Build history of the part. All positions in model axes, mm. Face numbers are marked on the shaded views. A direction names the side the tool comes from. Round coordinates to 2 decimals unless told otherwise and drop trailing zeros. Loops run counter-clockwise (first coordinate to the right, second up) from the corner with the lowest first, then second, coordinate; pieces in that order, holes last.
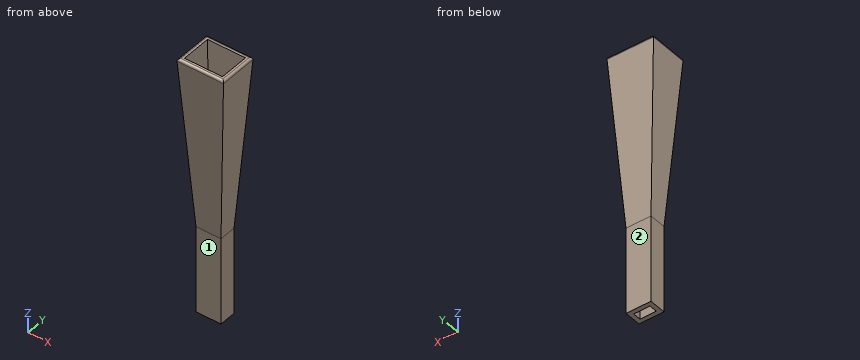
Autodesk Inventor part; units mm, degrees
ref_plane "Endebene" through (0, 0, 59.75) normal (0, 0, 1) x (1, 0, 0)
ref_plane "YZ Plane" through (0, 0, 0) normal (1, 0, 0) x (0, 1, 0)
ref_plane "XZ Plane" through (0, 0, 0) normal (0, 1, 0) x (-1, 0, 0)
sketch "Skizze1" plane through (0, 0, 0) normal (0, 0, 1) x (1, 0, 0)
  line L0 (1.8795, 0.94) -> (-1.8795, 0.94)
  line L1 (-1.8795, 0.94) -> (-1.8795, -0.94)
  line L2 (-1.8795, -0.94) -> (1.8795, -0.94)
  line L3 (1.8795, -0.94) -> (1.8795, 0.94)
  line L4 (1.8795, 0.94) -> (-1.8795, -0.94) construction
  line L5 (-1.8795, 0.94) -> (1.8795, -0.94) construction
  line L6 (-2.8795, -1.94) -> (-2.8795, 1.94)
  line L7 (-2.8795, 1.94) -> (2.8795, 1.94)
  line L8 (2.8795, 1.94) -> (2.8795, -1.94)
  line L9 (2.8795, -1.94) -> (-2.8795, -1.94)
  point P0 (0, 0)
  dimension "d0" = 1.88
  dimension "d1" = 3.759
  dimension "d2" = 1
extrude "Ex1-RWG" add sketch "Skizze1" along normal blind 20
ref_plane "Endebene" through (0, 0, 59.75) normal (0, 0, 1) x (1, 0, 0)
sketch "S-Hornöffnung" plane through (0, 0, 59.75) normal (0, 0, 1) x (1, 0, 0)
  line L0 (2.8795, -1.94) -> (2.8795, 1.94)
  line L1 (2.8795, 1.94) -> (-2.8795, 1.94)
  line L2 (-2.8795, 1.94) -> (-2.8795, -1.94)
  line L3 (-2.8795, -1.94) -> (2.8795, -1.94)
  line L4 (1.8795, 0.94) -> (1.8795, -0.94)
  line L5 (1.8795, -0.94) -> (-1.8795, -0.94)
  line L6 (-1.8795, -0.94) -> (-1.8795, 0.94)
  line L7 (-1.8795, 0.94) -> (1.8795, 0.94)
  line L8 (4.3795, 3.44) -> (4.3795, -3.44)
  line L9 (4.3795, -3.44) -> (-4.3795, -3.44)
  line L10 (-4.3795, -3.44) -> (-4.3795, 3.44)
  line L11 (-4.3795, 3.44) -> (4.3795, 3.44)
  line L12 (5.3795, -4.44) -> (5.3795, 4.44)
  line L13 (5.3795, 4.44) -> (-5.3795, 4.44)
  line L14 (-5.3795, 4.44) -> (-5.3795, -4.44)
  line L15 (-5.3795, -4.44) -> (5.3795, -4.44)
  point P0 (0, 0)
  dimension "d19" = 2.5
  dimension "d20" = 1
sketch "S-RWGÜbergang" plane through (0, 0, 20) normal (0, 0, 1) x (1, 0, 0)
  line L0 (2.8795, -1.94) -> (2.8795, 1.94)
  line L1 (2.8795, 1.94) -> (-2.8795, 1.94)
  line L2 (-2.8795, 1.94) -> (-2.8795, -1.94)
  line L3 (-2.8795, -1.94) -> (2.8795, -1.94)
  line L4 (1.8795, 0.94) -> (1.8795, -0.94)
  line L5 (1.8795, -0.94) -> (-1.8795, -0.94)
  line L6 (-1.8795, -0.94) -> (-1.8795, 0.94)
  line L7 (-1.8795, 0.94) -> (1.8795, 0.94)
  point P0 (0, 0)
loft "Erhebung-Horn1" add profiles "S-Hornöffnung" section 1 edges at (2.8795, 0, 20) (0, 1.94, 20) (-2.8795, 0, 20) (0, -1.94, 20) contours L3 L2 L1 L0 | L4 L5 L6 L7 | L8 L9 L10 L11 | L15 L14 L13 L12
loft "Erhebung-Horn2" cut profiles "S-Hornöffnung" section 1 edges at (0, 0.94, 20) (1.8795, 0, 20) (0, -0.94, 20) (-1.8795, 0, 20) contours L3 L2 L1 L0 | L4 L5 L6 L7 | L8 L9 L10 L11
fillet "Rundung-0.5mm" radius 0.5 4 edges at (0, 4.44, 59.75) (-5.3795, 0, 59.75) (0, -4.44, 59.75) (5.3795, 0, 59.75)
fillet_without_effect "Rundung-10mm"
properties part number "RWG_Horn_ProbeAntennaV1"
(1) Pin check, flat tips, straight feed: P1, Ø2, axis at y = 0, z = 5.5, coming from the +X side; P2, Ø2, axis at y = 1.5, z = 29.5, coming from the -X side; P3, Ø1.7, axis at x = 0, z = 11.5, coming from the -Y side. Stop position of each tip, or through.
Responses:
P1: stops at x = 2.88
P2: stops at x = -3.54
P3: stops at y = -1.94
(2) Which spindle directions (+Z, -Z, +X, -X, +Y, -Y) get a long thin tool onto all of the face, cutting with end or side? Do the marked faces 1 and 2. Say none if no direction does.
Responses:
face 1: -Z, +X, -X, -Y
face 2: -Z, +X, -X, +Y
(3) Probe line 1 (Y direction, x = -1, z = 35); line 2 (X direction, y = -1.5, z = 12); line 3 (X direction, y = 2, z = 41.5). List the from-to ranges inside material, lowest first.
Responses:
line 1: y = -2.88 to -1.88, 1.88 to 2.88
line 2: x = -2.88 to 2.88
line 3: x = -4.23 to -3.23, 3.23 to 4.23
(4) Slice it at A-A on z = 13. List the corners of the cut face in (x, y), plus the area to 3 significant figures.
Responses:
outline: (-2.88, -1.94) - (2.88, -1.94) - (2.88, 1.94) - (-2.88, 1.94) - close; hole (-1.88, -0.94) - (1.88, -0.94) - (1.88, 0.94) - (-1.88, 0.94) - close
area: 15.3 mm2
